Geometry check sheet. Reference: the model listing, model coordinates, mm. A direction names the side the tool comes from. Coordinates: 2 decimals unless noted, no trailing zeros. Order: outer loops, then holes, each group sorted by start corner. A loop starts at its lowest first (then second) coordinate and runs counter-clockwise, first axis right, second up. Notation, with made-up numbers: (3.25, 46.25) - (29.25, 46.25) arc R15 ccw to (29.25, 52.25) - close; hole circle Ø2 at (-11.75, 50.25). An arc over 180 degrees is marked (long way). Use CSV: the item, a comma, the result in double quotes. Start each with the question number.
1) Draft check along X on faces 1 (the flat face through (16.05, -4.14, 0)), 2 (the flat face through (-15.875, 0, -150)), 3 (the flat face through (-19.05, 0, -150)). Enter one of: released by +X, released by -X, zero draft, split by the parting line, or undercut.
2) Sectioned sample at C-C, the plane z = -78. Record the cut outline in (x, y) (3 decimals), and give its area (3 significant figures).
3) Thickness scan on probe 1 along X at (y, z) = (13, -67) (3 decimals); probe 2 along Y at (x, z) = (26, -246.5) (3 decimals). Record the ranges inside material, lowest first. Write a range as [from, to].
4) Sectioned sample at A-A, the plane x = -1. Record the cut outline in (y, z) (3 decimals), and give its area (3 significant figures).
5) Depth check by flat-ended pin: P1, Ø14.5, axis at y = 3.5, z = -141, coming from the +X side; P2, Ø1.5, axis at x = 19, z = -36, coming from the +Y side; P3, Ø6, axis at x = 26, z = -141, coming from the +Y side (3 decimals); P4, Ø4, axis at x = 23, y = 4.5, coming from the +Z side. Enter the tip coordinate at first touch or a pass-through.
6) Tool access check on faces 4 (the flat face through (0, -15.875, -150)), 5 (the flat face through (16.05, -4.14, -304.8)), 6 (the flat face through (39, -15.875, -150)). Record the directions out of +Z, -Z, +X, -X, +Y, -Y that give a thin tool (end or side, any length) a straight path to the whole face; none if there is none.
7) Sectioned sample at D-D, the plane x = 50. Record the cut outline in (y, z) (3 decimals).
Autodesk Inventor part; units mm, degrees
ref_plane "YZ Plane" through (0, 0, 0) normal (1, 0, 0) x (0, 1, 0)
ref_plane "XZ Plane" through (0, 0, 0) normal (0, 1, 0) x (-1, 0, 0)
ref_plane "XY Plane" through (0, 0, 0) normal (0, 0, 1) x (1, 0, 0)
sketch "Sketch1" plane through (0, 0, 0) normal (0, 0, 1) x (1, 0, 0)
  arc A0 (14.2748, -15.875) -> (15.875, -14.2748) centre (14.2748, -14.2748) ccw
  line L0 (15.875, -14.2748) -> (15.875, 14.2748)
  arc A1 (15.875, 14.2748) -> (14.2748, 15.875) centre (14.2748, 14.2748) ccw
  arc A2 (-14.2748, 15.875) -> (-15.875, 14.2748) centre (-14.2748, 14.2748) ccw
  line L1 (-15.875, 14.2748) -> (-15.875, -14.2748)
  arc A3 (-15.875, -14.2748) -> (-14.2748, -15.875) centre (-14.2748, -14.2748) ccw
  line L2 (-14.2748, -15.875) -> (14.2748, -15.875)
  line L3 (14.2748, 15.875) -> (-14.2748, 15.875)
  line L4 (-15.875, -19.05) -> (56.769, -19.05)
  line L5 (56.769, -19.05) -> (57.15, -18.669)
  line L6 (57.15, -18.669) -> (57.15, -16.256)
  line L7 (57.15, -16.256) -> (56.769, -15.875)
  line L8 (56.769, -15.875) -> (20.6502, -15.875)
  arc A4 (19.05, -14.2748) -> (20.6502, -15.875) centre (20.6502, -14.2748) ccw
  line L9 (19.05, -14.2748) -> (19.05, 15.875)
  arc A5 (19.05, 15.875) -> (15.875, 19.05) centre (15.875, 15.875) ccw
  line L10 (15.875, 19.05) -> (-15.875, 19.05)
  arc A6 (-15.875, 19.05) -> (-19.05, 15.875) centre (-15.875, 15.875) ccw
  line L11 (-19.05, 15.875) -> (-19.05, -15.875)
  arc A7 (-19.05, -15.875) -> (-15.875, -19.05) centre (-15.875, -15.875) ccw
  point P0 (0, 0)
extrude "Extrusion1" add sketch "Sketch1" against normal blind 304.8
properties part number "9705"
Evaluation:
1,face 1,"zero draft"
1,face 2,"undercut"
1,face 3,"released by -X"
2,outline,"(-19.05, -15.875) arc R3.175 ccw to (-15.875, -19.05) - (56.769, -19.05) - (57.15, -18.669) - (57.15, -16.256) - (56.769, -15.875) - (20.65, -15.875) arc R1.6 cw to (19.05, -14.275) - (19.05, 15.875) arc R3.175 ccw to (15.875, 19.05) - (-15.875, 19.05) arc R3.175 ccw to (-19.05, 15.875) - close; hole (-15.875, -14.275) arc R1.6 ccw to (-14.275, -15.875) - (14.275, -15.875) arc R1.6 ccw to (15.875, -14.275) - (15.875, 14.275) arc R1.6 ccw to (14.275, 15.875) - (-14.275, 15.875) arc R1.6 ccw to (-15.875, 14.275) - close"
2,area,"561 mm²"
3,probe 1,"[-19.05, -15.875], [15.875, 19.05]"
3,probe 2,"[-19.05, -15.875]"
4,outline,"(-19.05, -304.8) - (-15.875, -304.8) - (-15.875, 0) - (-19.05, 0) - close; (15.875, -304.8) - (19.05, -304.8) - (19.05, 0) - (15.875, 0) - close"
4,area,"1,940 mm²"
5,P1,"x = 19.05"
5,P2,"y = 17.98"
5,P3,"y = -15.875"
5,P4,"through"
6,face 4,"+Z, -Z"
6,face 5,"-Z, +X, -X, +Y, -Y"
6,face 6,"+Z, -Z, +X, +Y"
7,outline,"(-19.05, -304.8) - (-15.875, -304.8) - (-15.875, 0) - (-19.05, 0) - close"
